Build history of the part. All positions in model axes, mm. A direction names the side the tool comes from. Give positions to 0.01 mm unless a question says otherwise; leave off trailing zeros. Order: outer loops, then holes, each group sorted by start corner. A loop starts at its lowest first (then second) coordinate and runs counter-clockwise, first axis right, second up. Notation, with made-up numbers: (43, 61) - (59, 61) arc R18 cw to (59, 77) - close; hole circle Ø6 at (6.5, -3.5). An arc over 180 degrees is marked (long way). One line per item, written item: value.
```python
from build123d import *

# Parameters (mm, degrees)
SKETCH2_W           = 170
SKETCH2_H           = 5
BOSS_EXTRUDE1_DEPTH = 70


with BuildPart() as part:
    # Sketch2 → Boss-Extrude1 (new body)
    with BuildSketch(Plane(origin=(0, 0, 0), x_dir=(1, 0, 0), z_dir=(0, 1, 0))):
        with Locations((85, 2.5)):
            Rectangle(SKETCH2_W, SKETCH2_H)
        Polygon((-5, 0), (0, 0), (0, 5), (0, 32), (-5, 32), align=None)
    extrude(amount=BOSS_EXTRUDE1_DEPTH)


solid = part.part
```
(1) Slice it at A-A, the plane y = 58.5. Give the cut face in (x, z), and give its area (3 significant figures).
Completed:
outline: (-5, -32) - (0, -32) - (0, -5) - (170, -5) - (170, 0) - (-5, 0) - close
area: 1,010 mm²
(2) 3-axis set-ups, long thin cutter, end or side, ignore diameter. For faces 1 (the face through (0, 35, -18)), 2 (the face through (69, 70, -4)): which of +Z, -Z, +X, -X, +Y, -Y reach the whole face in a straight line?
Completed:
face 1: -Z, +X, +Y, -Y
face 2: +Z, -Z, +X, -X, +Y
(3) Drill centre line: line 1 (X direction, y = 45, z = -7). Where is it in solid material? Low to high.
Completed:
line 1: -5 to 0
(4) Slice it at B-B, the plane z = -9. Give the cut face in (x, y).
Completed:
outline: (-5, 0) - (0, 0) - (0, 70) - (-5, 70) - close
(5) Slice it at C-C, the plane x = 23.5. Give the cut face in (y, z).
Completed:
outline: (0, -5) - (70, -5) - (70, 0) - (0, 0) - close
(6) Pin check, flat tips, straight feed: P1, Ø4, axis at x = 73.5, y = 60, coming from the +Z side; P2, Ø8, axis at y = 46, z = -17.5, coming from the +X side; P3, Ø2, axis at x = 71, y = 18, coming from the -Z side. Stop position of each tip, or through.
Completed:
P1: z = 0
P2: x = 0
P3: z = -5
